Job drawing, mm, ordinate dimensions from the low corner. One solid piece. Coordinates: 2 decimals unless noted, no trailing zeros. Loops run counter-clockwise (first coordinate to the right, second up) from the corner with the lowest first, then second, coordinate; pieces in that order, holes last. Notation, with made-up numbers: (30, 33.25) -> (69, 33.25) arc R11 cw to (69, 48.25) -> close; hole circle Ø9 at (12, 84). An arc over 180 degrees is marked (long way). Answer as CSV lines item,"result". Start each with the question number.
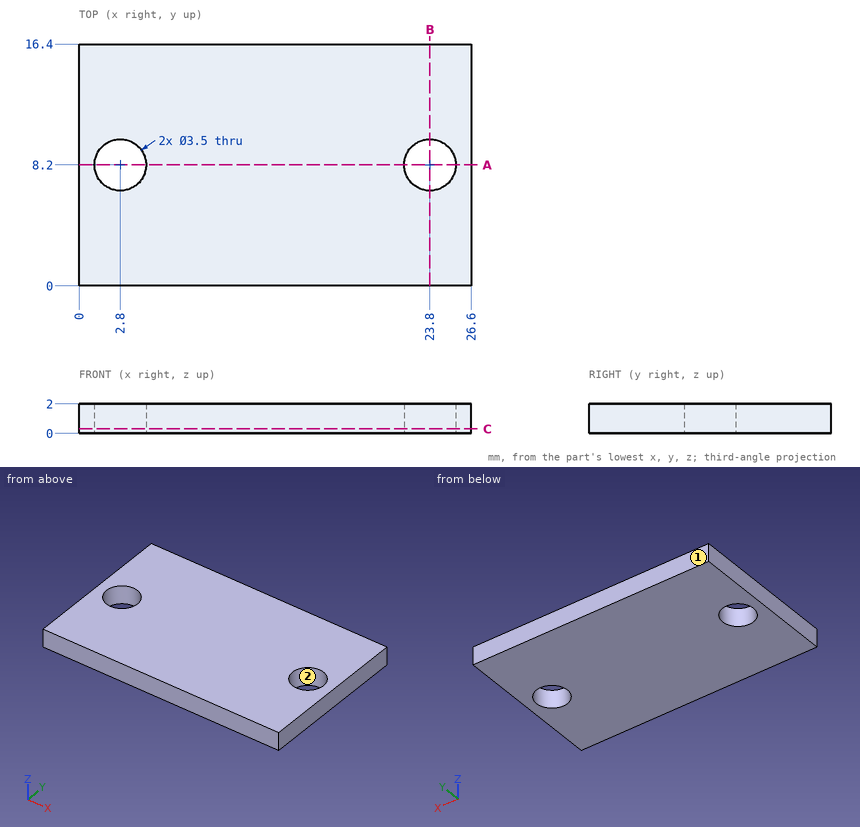
Q1. Saw through at A-A (y = 8.2). List the corners of the cut face in (x, z).
Q2. Two-plate mould, pull along X, no slides. Class the marked faces 1 and 2: pulls with the +X half, pulls with the -X half, needs draft (parallel to the pull), parting line crosses it, or undercut.
Q3. Saw through at B-B (x = 23.8). List the corners of the cut face in (y, z).
Q4. Probe probe 1 along X at (y, z) = (8.2, 0.95); probe 2 along Y at (x, z) = (23.8, 1.15). List the from-to ranges inside material, lowest first. Write a range as from..to.
Q5. Saw through at C-C (z = 0.3). List the corners of the cut face in (x, y).
Ans:
1,outline,"(0, 0) -> (1.05, 0) -> (1.05, 2) -> (0, 2) -> close; (4.55, 0) -> (22.05, 0) -> (22.05, 2) -> (4.55, 2) -> close; (25.55, 0) -> (26.6, 0) -> (26.6, 2) -> (25.55, 2) -> close"
2,face 1,"needs draft"
2,face 2,"undercut"
3,outline,"(0, 0) -> (6.45, 0) -> (6.45, 2) -> (0, 2) -> close; (9.95, 0) -> (16.4, 0) -> (16.4, 2) -> (9.95, 2) -> close"
4,probe 1,"x = 0..1.05, 4.55..22.05, 25.55..26.6"
4,probe 2,"y = 0..6.45, 9.95..16.4"
5,outline,"(0, 0) -> (26.6, 0) -> (26.6, 16.4) -> (0, 16.4) -> close; hole circle Ø3.5 at (2.8, 8.2); hole circle Ø3.5 at (23.8, 8.2)"
